Here's how the part is built. I have some questions about the finished solid (model axes, mm). A direction names the side the tool comes from. Coordinates: 2 decimals unless noted, no trailing zeros. Write each loop counter-clockwise with the first axis right and the second up, starting at its lowest first coordinate (ties: lowest second). Pieces come first, ordered by that corner, then holes.
```python
from build123d import *

# Parameters (mm, degrees)
BASE_EXTRUDE_DEPTH           = 121.285
SKETCH3_4_W                  = 12.658404279
SKETCH3_4_H                  = 69.85
MOTOR_BOX_CORE_SUPPORT_DEPTH = 172.085
WHEEL_SPACE_REACH            = 359.533
SKETCH4_W                    = 82.55
SKETCH4_H                    = 152.4
SKETCH5_W                    = 82.508404279
SKETCH5_H                    = 57.15
MOTOR_SPACE_DEPTH            = 121.285
MOTOR_SPACE_RIBS_DEPTH       = 358.532752856


with BuildPart() as part:
    # Sketch3 → Base extrude (new body)
    with BuildSketch(Plane(origin=(0, 0, 0), x_dir=(1, 0, 0), z_dir=(0, 1, 0))):
        with BuildLine():
            Line((26.55331123, 195.050875832), (28.266428083, 207.634803305))
            ThreePointArc((28.266428083, 207.634803305), (209.260756715, -11.006279992), (6.329202139, -209.454395276))
            Line((6.329202139, -209.454395276), (-6.329202139, -209.454395276))
            add(Edge.make_bspline(
                [(-146.008404279, -25.4), (-146.008404279, -25.825184703), (-146.008186701, -28.390264622), (-145.992828986, -37.675812079), (-145.847861717, -52.813230692), (-145.252148771, -71.571281929), (-144.048815033, -89.419368639), (-142.031880927, -106.362231784), (-137.954990072, -127.728726744), (-131.289734266, -147.26224301), (-120.928636207, -164.576629863), (-111.101066218, -176.207339111), (-99.137557526, -186.230706711), (-85.06323068, -194.472251254), (-71.591092365, -199.823977742), (-59.732617944, -203.218129468), (-50.280608969, -205.32790847), (-40.250071446, -207.008611147), (-31.389652459, -208.056286946), (-23.987147203, -208.684629614), (-18.276024056, -209.051283621), (-13.377371895, -209.269931643), (-9.381928102, -209.392630987), (-7.343469775, -209.4368391), (-6.329202139, -209.454395276)],
                knots=[0, 0, 0, 0, 0.003998364, 0.024104834, 0.088078657, 0.152052481, 0.216026304, 0.280000128, 0.343973951, 0.471921599, 0.535895422, 0.599869246, 0.663843069, 0.727816893, 0.791790716, 0.823777628, 0.85576454, 0.887751452, 0.919738363, 0.935731819, 0.951725275, 0.967718731, 0.975715459, 0.983712187, 0.983712187, 0.983712187, 0.983712187], degree=3))
            Line((-146.008404279, -25.4), (-133.35, -25.4))
            add(Edge.make_bspline(
                [(-133.35, -25.4), (-133.35, -131.233333333), (-127, -196.85), (0, -196.85)],
                knots=[0, 0, 0, 0, 1, 1, 1, 1], degree=3))
            ThreePointArc((0, -196.85), (196.39970393, -13.307095711), (26.55331123, 195.050875832))
        make_face()
    extrude(amount=BASE_EXTRUDE_DEPTH)

    # Sketch3<4> → Motor box & Core support (add)
    with BuildSketch(Plane(origin=(0, 0, 0), x_dir=(1, 0, 0), z_dir=(0, 1, 0))):
        with Locations((-139.67920214, 9.525)):
            Rectangle(SKETCH3_4_W, SKETCH3_4_H)
        with BuildLine():
            Line((-133.35, 44.45), (-133.35, -25.4))
            Line((-133.35, -25.4), (0, -25.4))
            ThreePointArc((0, -25.4), (24.821670104, -5.389312873), (10.533208363, 23.11301628))
            Line((10.533208363, 23.11301628), (-36.286529277, 44.45))
            Line((-36.286529277, 44.45), (-133.35, 44.45))
        make_face()
    extrude(amount=MOTOR_BOX_CORE_SUPPORT_DEPTH)

    # Sketch4 → Wheel space (cut, up to next)
    with BuildSketch(Plane.XY.offset(25.4), mode=Mode.PRIVATE) as wheel_space_sk1:
        with Locations((-15.875, 76.2)):
            Rectangle(SKETCH4_W, SKETCH4_H)
    wheel_space_tool1 = extrude(wheel_space_sk1.sketch, amount=-WHEEL_SPACE_REACH, mode=Mode.PRIVATE) & part.part
    add(wheel_space_tool1.solids().sort_by_distance((-15.875, 76.2, 25.4))[0], mode=Mode.SUBTRACT)

    # Sketch5 → Motor space (cut)
    with BuildSketch(Plane(origin=(0, 172.085, 0), x_dir=(1, 0, 0), z_dir=(0, 1, 0))):
        with Locations((-104.75420214, 9.525)):
            Rectangle(SKETCH5_W, SKETCH5_H)
    extrude(amount=-MOTOR_SPACE_DEPTH, mode=Mode.SUBTRACT)

    # Sketch6 → Motor Space Ribs (cut, through all)
    with BuildSketch(Plane.XY.offset(25.4)):
        Polygon((-146.008404279, 121.285), (-73.458485536, 172.085), (-146.008404279, 172.085), align=None)
    extrude(amount=-MOTOR_SPACE_RIBS_DEPTH, mode=Mode.SUBTRACT)


solid = part.part
```
1) Imagine slicing it at B-B on x = 65.5. Please give me the cut outline in (y, z) (3 decimals).
Values follow:
outline: (0, -199.05) - (121.285, -199.05) - (121.285, -185.633) - (0, -185.633) - close; (0, 185.633) - (121.285, 185.633) - (121.285, 199.05) - (0, 199.05) - close
2) Imagine slicing it at D-D on z = -181. Please give me the cut outline in (x, y) (3 decimals), then the cut area to 3 significant figures.
Values follow:
outline: (77.388, 0) - (105.595, 0) - (105.595, 121.285) - (77.388, 121.285) - close
area: 3,420 mm2
3) Imagine slicing it at A-A on z = 0. Please give me the cut outline in (x, y) (3 decimals), then the cut area to 3 significant figures.
Values follow:
outline: (-146.008, 0) - (-57.15, 0) - (-57.15, 152.4) - (25.4, 152.4) - (25.4, 172.085) - (-63.5, 172.085) - (-63.5, 50.8) - (-146.008, 50.8) - close; (196.85, 0) - (209.55, 0) - (209.55, 121.285) - (196.85, 121.285) - close
area: 8,450 mm2
4) On a 3-axis mill with a long thin cutter (end or side, diameter ignored), from which of +Z, -Z, +X, -X, +Y, -Y can I reach the whole of each face in a straight line? I mean faces 1 (the face through (-57.15, 75, -9)), 2 (the face through (-105, 50.8, -10)), 3 (the face through (-103, 85, -44.45)), 4 (the face through (196.076, 59.794, 17.437)), 5 (the face through (-26, 152.4, -1)). Say none if no direction works.
Values follow:
face 1: -Z, -Y
face 2: -X, +Y
face 3: -Z, -X, +Y, -Y
face 4: +Y, -Y
face 5: +Z, -Z, +X, -Y
5) I need wall thicknesses on probe 1 along Z at (x, y) = (-117, 110.5); probe 2 along Z at (x, y) = (-70.5, 88.5); probe 3 along Z at (x, y) = (-5.5, 112). Which ranges of each line are inside material? Lowest first, please.
Values follow:
probe 1: z = -44.45 to -38.1, 19.05 to 25.4, 145.88 to 169.04
probe 2: z = -44.45 to -38.1, 19.05 to 25.4, 186.51 to 199.95
probe 3: z = 196.81 to 209.45
6) Imagine slicing it at C-C on y = 134. Please give me the cut outline in (x, z), then the cut area to 3 significant figures.
Values follow:
outline: (-127.85, -44.45) - (-57.15, -44.45) - (-57.15, 25.4) - (-127.85, 25.4) - (-127.85, 19.05) - (-63.5, 19.05) - (-63.5, -38.1) - (-127.85, -38.1) - close
area: 1,260 mm2
7) Will these pins go through, and if not, where does the flat tip stop? pin 1 (6 mm diameter, centred on y = 58.5, z = -87.5, fed in from -X); pin 2 (8 mm diameter, centred on y = 82, z = -12, fed in from -X); pin 3 (6 mm diameter, centred on y = 117, z = 75, fed in from -X).
Values follow:
pin 1: stops at x = 174.81
pin 2: stops at x = -63.5
pin 3: stops at x = -145.12
8) We'd pull the mould along Z, two halves only. Please class faces 6 (the face through (-63.5, 112, -9)), 7 (the face through (-12.549, 162.105, -33.632)), 8 (the face through (209.445, 59.794, 6.645)): pulls with the +Z half, pulls with the -Z half, needs draft (parallel to the pull), parting line crosses it, or undercut.
Values follow:
face 6: undercut
face 7: pulls with the -Z half
face 8: parting line crosses it
